Could you check a few things on this model? Use its own coordinates, in mm. Face numbers are marked on the shaded views. A direction names the side the tool comes from. Coordinates: 2 decimals unless noted, no trailing zeros. Loops run counter-clockwise (first coordinate to the right, second up) from the corner with the lowest first, then second, coordinate; pieces in that order, holes last. Notation, with made-up numbers: (24, 32.5) - (52, 32.5) arc R19 ccw to (52, 69.5) - close; hole circle Ø11 at (60, -13.5). An arc over 180 degrees is marked (long way). Use CSV: the item, a comma, the result in double quotes.
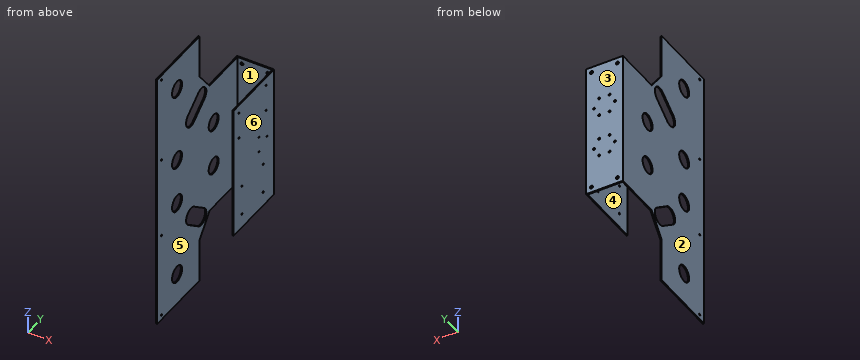
from build123d import *

# Parameters (mm, degrees)
BOSS_EXTRUDE1_DEPTH = 220
SKETCH2_R           = 1.7
CUT_EXTRUDE2_DEPTH  = 2
SKETCH3_R           = 1.15
CUT_EXTRUDE4_DEPTH  = 10
SKETCH4_R           = 1.5
CUT_EXTRUDE5_DEPTH  = 10
BOSS_EXTRUDE2_DEPTH = 2
SKETCH8_R           = 13.5
SKETCH8_R_2         = 1.5
CUT_EXTRUDE6_DEPTH  = 2
SKETCH9_R           = 2.5
CUT_EXTRUDE7_DEPTH  = 10


with BuildPart() as part:
    # Sketch1 → Boss-Extrude1 (new body)
    with BuildSketch(Plane.XY):
        Polygon((-58, -2), (-2, -2), (-2, -110), (0, -110), (0, 0), (-60, 0), (-60, -220), (-58, -220), align=None)
    extrude(amount=BOSS_EXTRUDE1_DEPTH)

    # Sketch2 → Cut-Extrude2 (cut)
    with BuildSketch(Plane(origin=(0, 0, 0), x_dir=(1, 0, 0), z_dir=(0, 1, 0))):
        with Locations(Location((-38.5, -59.777568136, 0), (0, 0, 270))):
            Circle(SKETCH2_R)
        with Locations(Location((-21.5, -59.777568136, 0), (0, 0, 270))):
            Circle(SKETCH2_R)
        with Locations(Location((-13, -74.5, 0), (0, 0, 270))):
            Circle(SKETCH2_R)
        with Locations(Location((-21.5, -89.222431864, 0), (0, 0, 270))):
            Circle(SKETCH2_R)
        with Locations(Location((-38.5, -89.222431864, 0), (0, 0, 270))):
            Circle(SKETCH2_R)
        with Locations(Location((-47, -74.5, 0), (0, 0, 270))):
            Circle(SKETCH2_R)
        with Locations(Location((-38.5, -130.777568136, 0), (0, 0, 270))):
            Circle(SKETCH2_R)
        with Locations(Location((-47, -145.5, 0), (0, 0, 270))):
            Circle(SKETCH2_R)
        with Locations(Location((-38.5, -160.222431864, 0), (0, 0, 270))):
            Circle(SKETCH2_R)
        with Locations(Location((-21.5, -160.222431864, 0), (0, 0, 270))):
            Circle(SKETCH2_R)
        with Locations(Location((-13, -145.5, 0), (0, 0, 270))):
            Circle(SKETCH2_R)
        with Locations(Location((-21.5, -130.777568136, 0), (0, 0, 270))):
            Circle(SKETCH2_R)
    extrude(amount=-CUT_EXTRUDE2_DEPTH, mode=Mode.SUBTRACT)

    # Sketch3 → Cut-Extrude4 (cut)
    with BuildSketch(Plane(origin=(0, 0, 0), x_dir=(0, 0, -1), z_dir=(1, 0, 0))):
        with Locations((-115, -19.001477372)):
            Circle(SKETCH3_R)
        with Locations((-127.7, -40.998522628)):
            Circle(SKETCH3_R)
        with Locations((-102.3, -40.998522628)):
            Circle(SKETCH3_R)
    extrude(amount=-CUT_EXTRUDE4_DEPTH, mode=Mode.SUBTRACT)

    # Sketch4 → Cut-Extrude5 (cut)
    with BuildSketch(Plane(origin=(0, 0, 0), x_dir=(0, 0, -1), z_dir=(1, 0, 0))):
        with Locations((-206.39781016, -21.433290156)):
            Circle(SKETCH4_R)
        with Locations((-162.39781016, -21.433290156)):
            Circle(SKETCH4_R)
        with Locations((-206.39781016, -95.433290156)):
            Circle(SKETCH4_R)
        with Locations((-162.39781016, -95.433290156)):
            Circle(SKETCH4_R)
        with Locations((-72.39781016, -29.433290156)):
            Circle(SKETCH4_R)
        with Locations((-23.39781016, -29.433290156)):
            Circle(SKETCH4_R)
        with Locations((-72.39781016, -87.433290156)):
            Circle(SKETCH4_R)
        with Locations((-23.39781016, -87.433290156)):
            Circle(SKETCH4_R)
    extrude(amount=-CUT_EXTRUDE5_DEPTH, mode=Mode.SUBTRACT)

    # Sketch6 → Boss-Extrude2 (add)
    with BuildSketch(Plane.ZY.offset(60)):
        Polygon((0, -78), (-34, -105), (-105, -105), (-105, -220), (0, -220), align=None)
        Polygon((220, -78), (220, -220), (325, -220), (325, -105), (254, -105), align=None)
    extrude(amount=-BOSS_EXTRUDE2_DEPTH)

    # Sketch8 → Cut-Extrude6 (cut)
    with BuildSketch(Plane.ZY.offset(60)):
        with Locations(Location((-53, -166, 0), (0, 0, 270))):
            Circle(SKETCH8_R)
        with Locations(Location((72, -166, 0), (0, 0, 270))):
            Circle(SKETCH8_R)
        with Locations(Location((148, -166, 0), (0, 0, 90))):
            Circle(SKETCH8_R)
        with Locations(Location((273, -166, 0), (0, 0, 90))):
            Circle(SKETCH8_R)
        with Locations(Location((-97.2, -208.2, 0), (0, 0, 270))):
            Circle(SKETCH8_R_2)
        with Locations(Location((43.5, -208.2, 0), (0, 0, 270))):
            Circle(SKETCH8_R_2)
        with Locations(Location((176.5, -208.2, 0), (0, 0, 90))):
            Circle(SKETCH8_R_2)
        with Locations(Location((317.2, -208.2, 0), (0, 0, 90))):
            Circle(SKETCH8_R_2)
        with Locations(Location((71.99, -66.8, 0), (0, 0, 270))):
            Circle(SKETCH8_R)
        with Locations(Location((148.01, -66.8, 0), (0, 0, 90))):
            Circle(SKETCH8_R)
        with BuildLine():
            Line((-7.563158771, -108.249005625), (13.500367039, -136.201248477))
            ThreePointArc((13.500367039, -136.201248477), (32.406449237, -138.85832505), (35.06352581, -119.952242852))
            Line((35.06352581, -119.952242852), (14, -92))
            ThreePointArc((14, -92), (-4.906082198, -89.342923427), (-7.563158771, -108.249005625))
        make_face()
        with BuildLine():
            Line((206, -92), (184.93647419, -119.952242852))
            ThreePointArc((184.93647419, -119.952242852), (187.593550763, -138.85832505), (206.499632961, -136.201248477))
            Line((206.499632961, -136.201248477), (227.563158771, -108.249005625))
            ThreePointArc((227.563158771, -108.249005625), (224.906082198, -89.342923427), (206, -92))
        make_face()
    extrude(amount=-CUT_EXTRUDE6_DEPTH, mode=Mode.SUBTRACT)

    # Sketch9 → Cut-Extrude7 (cut)
    with BuildSketch(Plane(origin=(0, 0, 0), x_dir=(1, 0, 0), z_dir=(0, 1, 0))):
        with Locations(Location((-51, -9, 0), (0, 0, 180))):
            Circle(SKETCH9_R)
        with Locations(Location((-9, -9, 0), (0, 0, 180))):
            Circle(SKETCH9_R)
        with Locations(Location((-9, -211, 0), (0, 0, 180))):
            Circle(SKETCH9_R)
        with Locations(Location((-51, -211, 0), (0, 0, 180))):
            Circle(SKETCH9_R)
    extrude(amount=-CUT_EXTRUDE7_DEPTH, mode=Mode.SUBTRACT)


solid = part.part
(1) Suppose I cut it at C-C (y = -172.5). Write out the boundary of the cut face in (x, z), plus the area to 3 significant figures.
Computed:
outline,"(-60, -105) - (-58, -105) - (-58, -64.83) - (-60, -64.83) - close; (-60, -41.17) - (-58, -41.17) - (-58, 60.17) - (-60, 60.17) - close; (-60, 83.83) - (-58, 83.83) - (-58, 136.17) - (-60, 136.17) - close; (-60, 159.83) - (-58, 159.83) - (-58, 261.17) - (-60, 261.17) - close; (-60, 284.83) - (-58, 284.83) - (-58, 325) - (-60, 325) - close"
area,"671 mm²"
(2) Suppose I cut it at D-D (z = -14.5). Write out the boundary of the cut face in (x, y), plus the area to 3 significant figures.
Computed:
outline,"(-60, -220) - (-58, -220) - (-58, -89.51) - (-60, -89.51) - close"
area,"261 mm²"
(3) Thinking about a two-plate mould opening in X: for the marked faces 1, 2, 3 and 4, which applies, +X half, -X half, draft (parallel to the pull), parting line (faces both ways), or undercut?
Computed:
face 1,"undercut"
face 2,"-X half"
face 3,"draft"
face 4,"undercut"
(4) Which directions (+Z, -Z, +X, -X, +Y, -Y) give clear straight access to the entire face, cutting with the end or side of a thin tool? Please do the marked faces 5 and 6.
Computed:
face 5,"+Z, -Z, -Y"
face 6,"+Z, -Z, +X, +Y, -Y"
(5) Suppose I cut it at A-A (z = 273). Write out the boundary of the cut face in (x, y), plus the area to 3 significant figures.
Computed:
outline,"(-60, -220) - (-58, -220) - (-58, -179.5) - (-60, -179.5) - close; (-60, -152.5) - (-58, -152.5) - (-58, -105) - (-60, -105) - close"
area,"176 mm²"
(6) Suppose I cut it at B-B (y = -132). Write out the boundary of the cut face in (x, z), plus the area to 3 significant figures.
Computed:
outline,"(-60, -105) - (-58, -105) - (-58, 10.33) - (-60, 10.33) - close; (-60, 37.2) - (-58, 37.2) - (-58, 182.8) - (-60, 182.8) - close; (-60, 209.67) - (-58, 209.67) - (-58, 325) - (-60, 325) - close"
area,"753 mm²"
(7) Please list where these lines run through material, in increasing order: line 1 (Z direction, x = -59, y = -208); line 2 (X direction, y = -1.2, z = 74.5); line 3 (X direction, y = -30, z = 168).
Computed:
line 1,"z = -105 to -98.69, -95.71 to 42.01, 44.99 to 175.01, 177.99 to 315.71, 318.69 to 325"
line 2,"x = -60 to -48.7, -45.3 to -14.7, -11.3 to 0"
line 3,"x = -60 to -58, -2 to 0"
(8) Will these pins go through, and if not, where does the flat tip stop? pin 1 (10 mm diameter, centred on y = -172, z = 153, fed in from +X); pin 2 (4.5 mm diameter, centred on x = -21.5, z = 160.22, fed in from -Y); pin 3 (4 mm diameter, centred on x = -21.5, z = 130.78, fed in from +Y); pin 4 (12 mm diameter, centred on y = -116.5, z = 0, fed in from +X).
Computed:
pin 1,"passes through"
pin 2,"stops at y = -2"
pin 3,"stops at y = 0"
pin 4,"stops at x = -58"
